Autodesk Inventor part; units mm, degrees
ref_plane "YZ Plane" through (0, 0, 0) normal (1, 0, 0) x (0, 1, 0)
ref_plane "XZ Plane" through (0, 0, 0) normal (0, 1, 0) x (-1, 0, 0)
ref_plane "XY Plane" through (0, 0, 0) normal (0, 0, 1) x (1, 0, 0)
sketch "草圖1" plane through (0, 0, 0) normal (0, 0, 1) x (1, 0, 0)
  line L0 (-2.5, -2.5) -> (2.5, -2.5)
  line L1 (2.5, -2.5) -> (2.5, 2.5)
  line L2 (2.5, 2.5) -> (-2.5, 2.5)
  line L3 (-2.5, 2.5) -> (-2.5, -2.5)
  line L4 (-2.5, -2.5) -> (2.5, 2.5) construction
  line L5 (2.5, -2.5) -> (-2.5, 2.5) construction
  arc A0 (-2.5, 2.5) -> (-2.5, -2.5) centre (-2.5, 0) ccw
  arc A1 (2.5, -2.5) -> (2.5, 2.5) centre (2.5, 0) ccw
  point P0 (0, 0)
  dimension "d0" = 5
  dimension "d1" = 5
extrude "擠出1" add sketch "草圖1" along normal blind 4
fillet "圓角1" radius 0.16 8 edges at (-5, 0, 4) (0, -2.5, 4) (5, 0, 4) (0, 2.5, 4) (5, 0, 0) (0, -2.5, 0) (-5, 0, 0) (0, 2.5, 0)
properties part number "key_3"
Read the model definition and answer for the solid it produces. Units are mm, in the model's axes. Round coordinates to 2 decimals unless told otherwise and drop trailing zeros. Write each loop counter-clockwise with the first axis right and the second up, starting at its lowest first coordinate (ties: lowest second). Pieces come first, ordered by that corner, then holes. Notation, with made-up numbers: (-2.75, -21) -> (18.25, -21) arc R22 ccw to (18.25, -4) -> close; hole circle Ø11 at (-19.5, -17). An arc over 180 degrees is marked (long way). Answer in a Markdown table with one row per item. Add a question column.
1) Find section A-A, the plane z = 0.45. Determine the outline of the cut face in (x, y), and give its area (3 significant figures).
2) Consider line 1 (X direction, y = -1.7, z = 0.9); line 2 (Y direction, x = -3.5, z = 3.4); line 3 (X direction, y = 0.8, z = 0.9). Determine where each line is inside the solid, lowest interval first.
3) Given P1, Ø1.5, axis at y = -1.5, z = 3.5, coming from the -X side, flat-ended and moving along its own axis, determine where the tip first touches the part or whether it passes through.
Findings below:
| question | item | result |
|---|---|---|
| 1 | outline | (-2.5, -2.5) -> (2.5, -2.5) arc R2.5 ccw to (2.5, 2.5) -> (-2.5, 2.5) arc R2.5 ccw to start |
| 1 | area | 44.6 mm² |
| 2 | line 1 | -4.33 to 4.33 |
| 2 | line 2 | -2.29 to 2.29 |
| 2 | line 3 | -4.87 to 4.87 |
| 3 | P1 | x = -4.88 |
